```python
from build123d import *

# Parameters (mm, degrees)
SKETCH1_W                = 155.575
SKETCH1_H                = 107.237500028
BOSS_EXTRUDE1_DEPTH      = 36.5
SHELL2_T                 = -3.175
FILLET1_R                = 2.54
CUT_EXTRUDE2_REACH       = 194.447
SKETCH7_R                = 1.2
SKETCH7_W                = 15
SKETCH7_H                = 15
SKETCH8_R                = 2.38125
CUT_EXTRUDE3_DEPTH       = 190.889155594
M3_CLEARANCE_HOLE1_D     = 3.4
M3_CLEARANCE_HOLE1_DEPTH = 3.175


with BuildPart() as part:
    # Sketch1 → Boss-Extrude1 (new body)
    with BuildSketch(Plane(origin=(0, 0, 0), x_dir=(0, 0, -1), z_dir=(1, 0, 0))):
        with Locations((77.7875, 53.618750014)):
            Rectangle(SKETCH1_W, SKETCH1_H)
    extrude(amount=BOSS_EXTRUDE1_DEPTH)

    # Shell2
    shell2_openings = [part.faces().sort_by_distance(p)[0] for p in [
        (18.25, 53.618750014, 0),
    ]]
    offset(amount=SHELL2_T, openings=shell2_openings, kind=Kind.INTERSECTION)

    # Fillet1
    fillet1_edges = [part.edges().sort_by_distance(p)[0] for p in [
        (36.5, 107.237500028, -77.7875),
        (0, 107.237500028, -77.7875),
        (0, 0, -77.7875),
        (36.5, 0, -77.7875),
    ]]
    fillet(fillet1_edges, radius=FILLET1_R)

    # Sketch7 → Cut-Extrude2 (cut, up to next)
    with BuildSketch(Plane(origin=(0, 0, -155.575), x_dir=(-1, 0, 0), z_dir=(0, 0, -1)), mode=Mode.PRIVATE) as cut_extrude2_sk1:
        with Locations((-7.175, 30)):
            Circle(SKETCH7_R)
    cut_extrude2_tool1 = extrude(cut_extrude2_sk1.sketch, amount=-CUT_EXTRUDE2_REACH, mode=Mode.PRIVATE) & part.part
    # Sketch7 → Cut-Extrude2 (cut, up to next)
    with BuildSketch(Plane(origin=(0, 0, -155.575), x_dir=(-1, 0, 0), z_dir=(0, 0, -1)), mode=Mode.PRIVATE) as cut_extrude2_sk2:
        with Locations((-7.175, 5)):
            Circle(SKETCH7_R)
    cut_extrude2_tool2 = extrude(cut_extrude2_sk2.sketch, amount=-CUT_EXTRUDE2_REACH, mode=Mode.PRIVATE) & part.part
    # Sketch7 → Cut-Extrude2 (cut, up to next)
    with BuildSketch(Plane(origin=(0, 0, -155.575), x_dir=(-1, 0, 0), z_dir=(0, 0, -1)), mode=Mode.PRIVATE) as cut_extrude2_sk3:
        with Locations((-20.675, 27.5)):
            Rectangle(SKETCH7_W, SKETCH7_H)
    cut_extrude2_tool3 = extrude(cut_extrude2_sk3.sketch, amount=-CUT_EXTRUDE2_REACH, mode=Mode.PRIVATE) & part.part
    add(cut_extrude2_tool1.solids().sort_by_distance((7.175, 30, -155.575))[0], mode=Mode.SUBTRACT)
    add(cut_extrude2_tool2.solids().sort_by_distance((7.175, 5, -155.575))[0], mode=Mode.SUBTRACT)
    add(cut_extrude2_tool3.solids().sort_by_distance((20.675, 27.5, -155.575))[0], mode=Mode.SUBTRACT)

    # Sketch8 → Cut-Extrude3 (cut, through all)
    with BuildSketch(Plane.XY.offset(-152.4)):
        with Locations((7.175, 25.4)):
            Circle(SKETCH8_R)
    extrude(amount=-CUT_EXTRUDE3_DEPTH, mode=Mode.SUBTRACT)

    # M3 Clearance Hole1
    with Locations(Plane(origin=(36.5, 0, 0), x_dir=(0, 0, -1), z_dir=(1, 0, 0))):
        with Locations((144.7875, 86.618750014), (144.7875, 20.618750014), (10.7875, 6.618750014), (10.7875, 100.618750014)):
            Hole(M3_CLEARANCE_HOLE1_D / 2, depth=M3_CLEARANCE_HOLE1_DEPTH)


solid = part.part
```
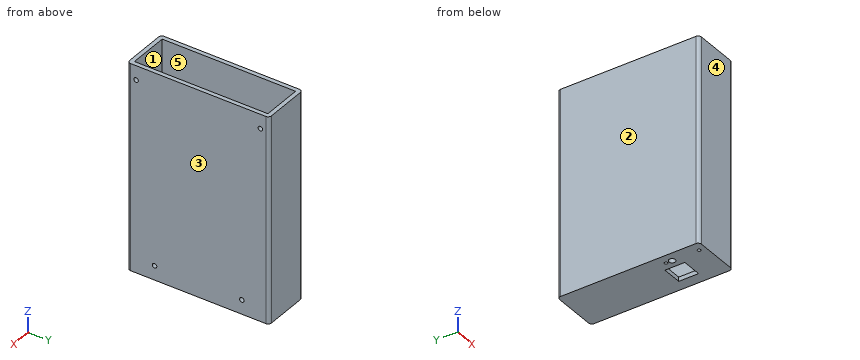
Verification items for the finished model (mm, model axes). Face numbers are marked on the shaded views. A direction names the side the tool comes from. Give positions to 0.01 mm unless a question says otherwise; leave off trailing zeros. Order: outer loops, then holes, each group sorted by start corner. A loop starts at its lowest first (then second) coordinate and runs counter-clockwise, first axis right, second up. Notation, with made-up numbers: M 0,79.25 L 14,79.25 A29 ccw 14,111.25 Z; hole C 68.5,27.25 d5. An arc over 180 degrees is marked long. Answer in a Markdown table with one row per item. Add a question column.
Item 1: Section check B-B, the plane y = 38. Enter the section's corners in (x, z) (3 decimals).
Item 2: Scan lines: probe 1 along X at (y, z) = (8.5, -136) (3 decimals); probe 2 along Y at (x, z) = (28, -12.5) (1 decimal); probe 3 along Z at (x, y) = (32, 18.5) (3 decimals). Record each from-to range of solid material in increasing order. Write a range as from..to.
Item 3: Gauge pin test, flat ends, axial feed: pin 1 (2 mm diameter, centred on x = 7.175, y = 5, fed in from -Z); pin 2 (3 mm diameter, centred on y = 100.62, z = -10.79, fed in from +X) (3 decimals); pin 3 (1.5 mm diameter, centred on x = 15.5, y = 43, fed in from +Z). Record the tip position at first contact, or that the pin passes through.
Item 4: Section check A-A, the plane z = -111. Enter the section's corners in (x, y) (1 decimal).
Item 5: Tool access check on the marked faces 1 and 2. Record the directions out of +Z, -Z, +X, -X, +Y, -Y that give a thin tool (end or side, any length) a straight path to the whole face; none if there is none.
Item 6: Mould release check, pull along Y, two halves, no side actions. Record for the marked faces 3, 4 and 5: released by +Y, released by -Y, zero draft, split by the parting line, or undercut.
Filled sheet:
| question | item | result |
|---|---|---|
| 1 | outline | M 0,-155.575 L 36.5,-155.575 L 36.5,0 L 33.325,0 L 33.325,-152.4 L 3.175,-152.4 L 3.175,0 L 0,0 Z |
| 2 | probe 1 | x = 0..3.175, 33.325..36.5 |
| 2 | probe 2 | y = 0..3.2, 104.1..107.2 |
| 2 | probe 3 | z = -155.575..-152.4 |
| 3 | pin 1 | passes through |
| 3 | pin 2 | stops at x = 3.175 |
| 3 | pin 3 | stops at z = -152.4 |
| 4 | outline | M 0,2.5 A2.5 ccw 2.5,0 L 34,0 A2.5 ccw 36.5,2.5 L 36.5,104.7 A2.5 ccw 34,107.2 L 2.5,107.2 A2.5 ccw 0,104.7 Z; hole M 3.2,3.2 L 33.3,3.2 L 33.3,104.1 L 3.2,104.1 Z |
| 5 | face 1 | +Z |
| 5 | face 2 | +Z, -Z, -X, +Y, -Y |
| 6 | face 3 | zero draft |
| 6 | face 4 | released by -Y |
| 6 | face 5 | undercut |
